For this review, take the finished solid that the model builds, in its own axes (mm). Face numbers are marked on the shaded views. A direction names the side the tool comes from. Give positions to 0.01 mm unless a question says otherwise; leave off trailing zeros. Write each loop counter-clockwise with the first axis right and the second up, starting at its lowest first coordinate (ties: lowest second). Pieces come first, ordered by that corner, then holes.
1) We need section A-A on y = -1. Give the boundary of the cut face in (x, z), and give its area (3 significant figures).
2) We need section D-D on y = 3.5. Give the number of separate pieces and of enclosed holes in the cut face, and give its area (3 significant figures).
3) Wall thickness on line 1 along Z through (x, y) = (8, 3.5); line 2 along X through (y, z) = (3.75, 3.5); line 3 along X through (y, z) = (0.25, 9): over which ranges is each line inside the solid? List them lowest first.
4) We need section B-B on x = 14. Give the boundary of the cut face in (y, z).
5) Machinability: for the marked faces 1 and 2, which of the approach directions +Z, -Z, +X, -X, +Y, -Y give a long, thin tool a straight path to every point of the face, cutting with its end or side? Answer none if there is none.
6) We need section C-C on z = 1. Give the boundary of the cut face in (x, y).
7) For P1, Ø4, axis at x = 8, z = 10.5, coming from the -Y side; P2, Ø1, axis at y = -2.5, z = 7, coming from the -X side; P3, Ø3, axis at x = 3, y = -2, coming from the -Z side; P4, Ø0.5, axis at y = 4, z = 8.5, coming from the +X side, all flat-tipped, find the tip position at first contact; note any pin that passes through.
from build123d import *

# Parameters (mm, degrees)
SKETCH1_W           = 15.5
SKETCH1_H           = 12
BOSS_EXTRUDE1_DEPTH = 5.5
SKETCH2_W           = 0.5
SKETCH2_H           = 0.5
BOSS_EXTRUDE2_DEPTH = 0.7
SKETCH3_W           = 0.5
SKETCH3_H           = 0.5
BOSS_EXTRUDE3_DEPTH = 6
SKETCH4_W           = 1
SKETCH4_H           = 1
CUT_EXTRUDE1_DEPTH  = 3
LPATTERN1_COUNT     = 5
LPATTERN1_PITCH     = 2
FILLET1_R           = 0.2
FILLET2_R           = 0.2


with BuildPart() as part:
    # Sketch1 → Boss-Extrude1 (new body)
    with BuildSketch(Plane(origin=(0, 0, 0), x_dir=(1, 0, 0), z_dir=(0, 1, 0))):
        with Locations((7.75, -6)):
            Rectangle(SKETCH1_W, SKETCH1_H)
    extrude(amount=BOSS_EXTRUDE1_DEPTH)

    # Sketch2 → Boss-Extrude2 (add)
    with BuildSketch(Plane(origin=(15.5, 0, 0), x_dir=(0, 0, -1), z_dir=(1, 0, 0))):
        with Locations((-9.81, 2.75)):
            Rectangle(SKETCH2_W, SKETCH2_H)
        with Locations((-7.27, 2.75)):
            Rectangle(SKETCH2_W, SKETCH2_H)
        with Locations((-4.73, 2.75)):
            Rectangle(SKETCH2_W, SKETCH2_H)
        with Locations((-2.19, 2.75)):
            Rectangle(SKETCH2_W, SKETCH2_H)
    extrude(amount=BOSS_EXTRUDE2_DEPTH)

    # Sketch3 → Boss-Extrude3 (add)
    with BuildSketch(Plane.XZ.offset(-2.5)):
        with Locations((15.95, 9.81)):
            Rectangle(SKETCH3_W, SKETCH3_H)
        with Locations((15.95, 7.27)):
            Rectangle(SKETCH3_W, SKETCH3_H)
        with Locations((15.95, 4.73)):
            Rectangle(SKETCH3_W, SKETCH3_H)
        with Locations((15.95, 2.19)):
            Rectangle(SKETCH3_W, SKETCH3_H)
    extrude(amount=BOSS_EXTRUDE3_DEPTH)

    # Sketch4 → Cut-Extrude1 (cut)
    with BuildSketch(Plane(origin=(0, 5.5, 0), x_dir=(1, 0, 0), z_dir=(0, 1, 0))):
        with Locations((2.281693228, -3.5)):
            Rectangle(SKETCH4_W, SKETCH4_H)
        with Locations((2.281693228, -6)):
            Rectangle(SKETCH4_W, SKETCH4_H)
        with Locations((2.281693228, -8.5)):
            Rectangle(SKETCH4_W, SKETCH4_H)
    cut_extrude1 = extrude(amount=-CUT_EXTRUDE1_DEPTH, mode=Mode.SUBTRACT)

    # LPattern1: Cut-Extrude1 ×5
    with Locations(*[(i * LPATTERN1_PITCH, 0, 0) for i in range(1, LPATTERN1_COUNT)]):
        add(cut_extrude1, mode=Mode.SUBTRACT)

    # Fillet1
    fillet1_edges = [part.edges().sort_by_distance(p)[0] for p in [
        (2.781693228, 5.5, 3.5),
        (2.281693228, 5.5, 3),
        (1.781693228, 5.5, 3.5),
        (2.281693228, 5.5, 4),
        (15.5, 5.5, 6),
        (1.781693228, 5.5, 6),
        (2.281693228, 5.5, 6.5),
        (2.781693228, 5.5, 6),
        (2.281693228, 5.5, 5.5),
        (1.781693228, 5.5, 8.5),
        (2.281693228, 5.5, 9),
        (2.781693228, 5.5, 8.5),
        (2.281693228, 5.5, 8),
        (4.781693228, 5.5, 3.5),
        (4.281693228, 5.5, 3),
        (3.781693228, 5.5, 3.5),
        (4.281693228, 5.5, 4),
        (6.781693228, 5.5, 3.5),
        (7.75, 5.5, 0),
        (6.281693228, 5.5, 4),
        (5.781693228, 5.5, 3.5),
        (6.281693228, 5.5, 3),
        (8.781693228, 5.5, 3.5),
        (8.281693228, 5.5, 4),
        (7.781693228, 5.5, 3.5),
        (8.281693228, 5.5, 3),
        (10.781693228, 5.5, 3.5),
        (10.281693228, 5.5, 4),
        (9.781693228, 5.5, 3.5),
        (10.281693228, 5.5, 3),
        (3.781693228, 5.5, 8.5),
        (4.281693228, 5.5, 9),
        (4.781693228, 5.5, 8.5),
        (4.281693228, 5.5, 8),
        (5.781693228, 5.5, 8.5),
        (6.281693228, 5.5, 8),
        (6.781693228, 5.5, 8.5),
        (6.281693228, 5.5, 9),
        (7.781693228, 5.5, 8.5),
        (8.281693228, 5.5, 8),
        (8.781693228, 5.5, 8.5),
        (8.281693228, 5.5, 9),
        (9.781693228, 5.5, 8.5),
        (10.281693228, 5.5, 8),
        (10.781693228, 5.5, 8.5),
        (10.281693228, 5.5, 9),
        (3.781693228, 5.5, 6),
        (4.281693228, 5.5, 6.5),
        (4.781693228, 5.5, 6),
        (4.281693228, 5.5, 5.5),
        (5.781693228, 5.5, 6),
        (6.281693228, 5.5, 5.5),
        (6.781693228, 5.5, 6),
        (6.281693228, 5.5, 6.5),
        (7.781693228, 5.5, 6),
        (8.281693228, 5.5, 5.5),
        (8.781693228, 5.5, 6),
        (8.281693228, 5.5, 6.5),
        (9.781693228, 5.5, 6),
        (10.281693228, 5.5, 5.5),
        (10.781693228, 5.5, 6),
        (10.281693228, 5.5, 6.5),
        (0, 5.5, 6),
        (7.75, 5.5, 12),
    ]]
    fillet(fillet1_edges, radius=FILLET1_R)

    # Fillet2
    fillet2_edges = [part.edges().sort_by_distance(p)[0] for p in [
        (7.75, 0, 0),
        (15.5, 0, 6),
        (7.75, 0, 12),
        (0, 0, 6),
    ]]
    fillet(fillet2_edges, radius=FILLET2_R)


solid = part.part
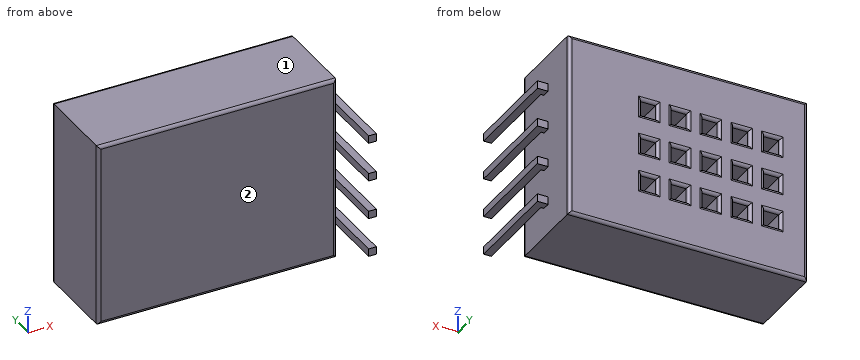
Results list:
1. outline: (15.7, 1.94) - (16.2, 1.94) - (16.2, 2.44) - (15.7, 2.44) - close; (15.7, 4.48) - (16.2, 4.48) - (16.2, 4.98) - (15.7, 4.98) - close; (15.7, 7.02) - (16.2, 7.02) - (16.2, 7.52) - (15.7, 7.52) - close; (15.7, 9.56) - (16.2, 9.56) - (16.2, 10.06) - (15.7, 10.06) - close
1. area: 1.00 mm2
2. separate pieces: 1
2. enclosed holes: 15
2. area: 171 mm2
3. line 1: z = 0 to 3, 4 to 5.5, 6.5 to 8, 9 to 12
3. line 2: x = 0 to 1.78, 2.78 to 3.78, 4.78 to 5.78, 6.78 to 7.78, 8.78 to 9.78, 10.78 to 15.5
3. line 3: x = 0 to 15.5
4. outline: (0, 0.2) arc R0.2 ccw to (0.2, 0) - (5.3, 0) arc R0.2 ccw to (5.5, 0.2) - (5.5, 11.8) arc R0.2 ccw to (5.3, 12) - (0.2, 12) arc R0.2 ccw to (0, 11.8) - close
5. face 1: +Z, +X, -X, +Y, -Y
5. face 2: +Z, -Z, -X, -Y
6. outline: (0, 0.2) arc R0.2 ccw to (0.2, 0) - (15.3, 0) arc R0.2 ccw to (15.5, 0.2) - (15.5, 5.3) arc R0.2 ccw to (15.3, 5.5) - (0.2, 5.5) arc R0.2 ccw to (0, 5.3) - close
7. P1: stops at y = 0
7. P2: stops at x = 15.7
7. P3: passes through
7. P4: stops at x = 15.5
